```python
from build123d import *

# Parameters (mm, degrees)
SKETCH_1_R      = 1.65
EXTRUDE_1_DEPTH = 5
FILLET_2_R      = 4
FILLET_3_R      = 40
FILLET_4_R      = 10


with BuildPart() as part:
    # 草图1 → 凸台-拉伸1 (new body)
    with BuildSketch(Plane.XY):
        with BuildLine():
            Line((-11.5, 79.5), (-11.5, 82))
            ThreePointArc((-11.5, 82), (6.103622298, 73.512939805), (10.426977744, 54.454442843))
            Line((10.426977744, 54.454442843), (13.41461423, 33.96926032))
            Line((13.41461423, 33.96926032), (11.539893904, 12.741041785))
            Line((11.539893904, 12.741041785), (4.278741136, 12.025251419))
            Line((4.278741136, 12.025251419), (-1.047111461, 14.664575003))
            Line((-1.047111461, 14.664575003), (3.709660575, 42.919402146))
            ThreePointArc((3.709660575, 42.919402146), (-2.22232543, 39.001835337), (-9.080443962, 37.130472768))
            Line((-9.080443962, 37.130472768), (-9.349283522, 39.615975794))
            ThreePointArc((-9.349283522, 39.615975794), (8.470985005, 60.576920581), (-11.5, 79.5))
        make_face()
        with Locations((5.679475492, 16.683750627)):
            Circle(SKETCH_1_R, mode=Mode.SUBTRACT)
        with Locations((8.382327473, 29.399669437)):
            Circle(SKETCH_1_R, mode=Mode.SUBTRACT)
    extrude(amount=EXTRUDE_1_DEPTH)

    # 圆角2
    fillet_2_edges = [part.edges().sort_by_distance(p)[0] for p in [
        (10.426977744, 54.454442843, 2.5),
    ]]
    fillet(fillet_2_edges, radius=FILLET_2_R)

    # 圆角3
    fillet_3_edges = [part.edges().sort_by_distance(p)[0] for p in [
        (13.41461423, 33.96926032, 2.5),
    ]]
    fillet(fillet_3_edges, radius=FILLET_3_R)

    # 圆角4
    fillet_4_edges = [part.edges().sort_by_distance(p)[0] for p in [
        (4.278741136, 12.025251419, 2.5),
    ]]
    fillet(fillet_4_edges, radius=FILLET_4_R)


solid = part.part
```
Could you check a few things on this model? Use its own coordinates, in mm. A direction names the side the tool comes from. Round coordinates to 2 decimals unless told otherwise and drop trailing zeros. Write each loop counter-clockwise with the first axis right and the second up, starting at its lowest first coordinate (ties: lowest second). Pieces come first, ordered by that corner, then holes. Notation, with made-up numbers: M 76,-29 L 90,-29 A23 cw 90,-20 Z; hole C 75,24.25 d9. An arc over 180 degrees is marked long. Answer in a Markdown table with one row per item. Add a question column.
Q1. On a 3-axis mill with a long thin cutter (end or side, diameter ignored), from which of +Z, -Z, +X, -X, +Y, -Y can I reach the whole of each face in a straight line? I mean faces 4 (the flat face through (11.62, 46.28, 2.46)), 5 (the flat face through (-9.213, 38.356, 2.465)), 6 (the flat face through (1.3, 28.6, 2.5)). Say none if no direction works.
Q2. Imagine slicing it at D-D (x = 0). Please give me the cut outline in (y, z).
Q3. Imagine slicing it at C-C (y = 41). Please give me the cut outline in (x, z).
Q4. Imagine slicing it at A-A (x = -5.5). Please give me the cut outline in (y, z), then the cut area to 3 significant figures.
Q5. If I drill on line 1 (Y direction, x = 4.25, z = 1.2); line 2 (Y direction, x = -6, z = 0.2); line 3 (Y direction, x = -4.75, z = 0.45), over which ranges is the centre line in solid material (lowest first)? Write a range as from..to.
Q6. Will these pins go through, and if not, where does the flat tip stop? pin 1 Ø1.5 at (y, z) = (23, 3) entering from +X; pin 2 Ø3 at (y, z) = (57.5, 2) entering from -X; pin 3 Ø2 at (y, z) = (71.5, 1) entering from +X.
Q7. Imagine slicing it at B-B (z = 2). Please give me the cut outline in (x, y).
Q8. If we mould it in two halves opening along X, with no side actions, what happens to faces 1 (the flat face through (6, 40, 0)), 2 (the cylindrical face through (5.322, 15.073, 2.465)), 3 (the cylindrical face through (10.49, 54.43, 2.54))? For each: +X half, -X half, draft (parallel to the pull), parting line (faces both ways), or undercut.
Values:
| question | item | result |
|---|---|---|
| 1 | face 4 | +Z, -Z, +X |
| 1 | face 5 | +Z, -Z, -X, -Y |
| 1 | face 6 | +Z, -Z |
| 2 | outline | M 14.15,0 L 20.88,0 L 20.88,5 L 14.15,5 Z; M 40.16,0 L 43.14,0 L 43.14,5 L 40.16,5 Z; M 75.86,0 L 78.84,0 L 78.84,5 L 75.86,5 Z |
| 3 | outline | M -3.9,0 L 1.31,0 L 1.31,5 L -3.9,5 Z; M 3.39,0 L 12.39,0 L 12.39,5 L 3.39,5 Z |
| 4 | outline | M 37.81,0 L 40.42,0 L 40.42,5 L 37.81,5 Z; M 78.58,0 L 81.19,0 L 81.19,5 L 78.58,5 Z |
| 4 | area | 26.1 mm^2 |
| 5 | line 1 | 12.44..15.86, 17.51..47.17, 71.83..75.57 |
| 5 | line 2 | 37.68..40.27, 78.73..81.32 |
| 5 | line 3 | 38.04..40.67, 78.33..80.96 |
| 6 | pin 1 | x = 12.51 |
| 6 | pin 2 | x = 8.19 |
| 6 | pin 3 | x = 8.13 |
| 7 | outline | M -11.5,79.5 A20 cw -9.35,39.62 L -9.08,37.13 A22.5 ccw 3.71,42.92 L -1.05,14.66 L 1.71,13.3 A10 ccw 7.13,12.31 L 11.54,12.74 L 13,29.31 A40 ccw 12.74,38.6 L 10.53,53.74 A4 cw 10.57,55.1 A22.5 ccw -11.5,82 Z; hole C 5.68,16.68 d3.3; hole C 8.38,29.4 d3.3 |
| 8 | face 1 | draft |
| 8 | face 2 | undercut |
| 8 | face 3 | +X half |
